Job drawing, mm, ordinate dimensions from the low corner. One solid piece. A direction names the side the tool comes from. Coordinates: 2 decimals unless noted, no trailing zeros. Order: outer loops, then holes, each group sorted by start corner. A loop starts at its lowest first (then second) coordinate and runs counter-clockwise, first axis right, second up. Notation, with made-up numbers: (-27.5, 32.25) - (-2.5, 32.25) arc R36 ccw to (-2.5, 70.25) - close; hole circle Ø7 at (-6, -36). An arc over 180 degrees is marked (long way). Use a Markdown table: item, result. Add a question column.
1) Saw through at A-A on z = 9.5. List the corners of the cut face in (x, y), then the cut area to 3 significant figures.
2) Wall check: L1, parallel to X at y = 0.7, z = 10; L2, parallel to X at y = 0.9, z = 9.5; L3, parallel to Z at x = 32.5, y = 2.25. Give the ranges that are in metal, low to high. Write a range as [from, to].
3) Two-plate mould, pull along Z, no slides. Class the marked faces 1, 2, 3 and 4: +Z half, -Z half, draft (parallel to the pull), parting line (faces both ways), or undercut.
4) Drop flat-ended pins along their axis: P1, Ø1.9, axis at x = 13, z = 24, coming from the +Y side; P2, Ø1, axis at y = 0.5, z = 23.5, coming from the -X side. Give the stop position or say it passes through.
5) Saw through at B-B on x = 13. List the corners of the cut face in (y, z).
6) Saw through at D-D on x = 28. List the corners of the cut face in (y, z).
7) Saw through at C-C on y = 1.9. Count the separate pieces of the cut face and the enclosed holes in it, then the cut area to 3 significant figures.
8) Tool access for the marked faces 5, 6 and 7: list every direction of +Z, -Z, +X, -X, +Y, -Y with a clear straight run to the whole face (end or side of a thin tool).
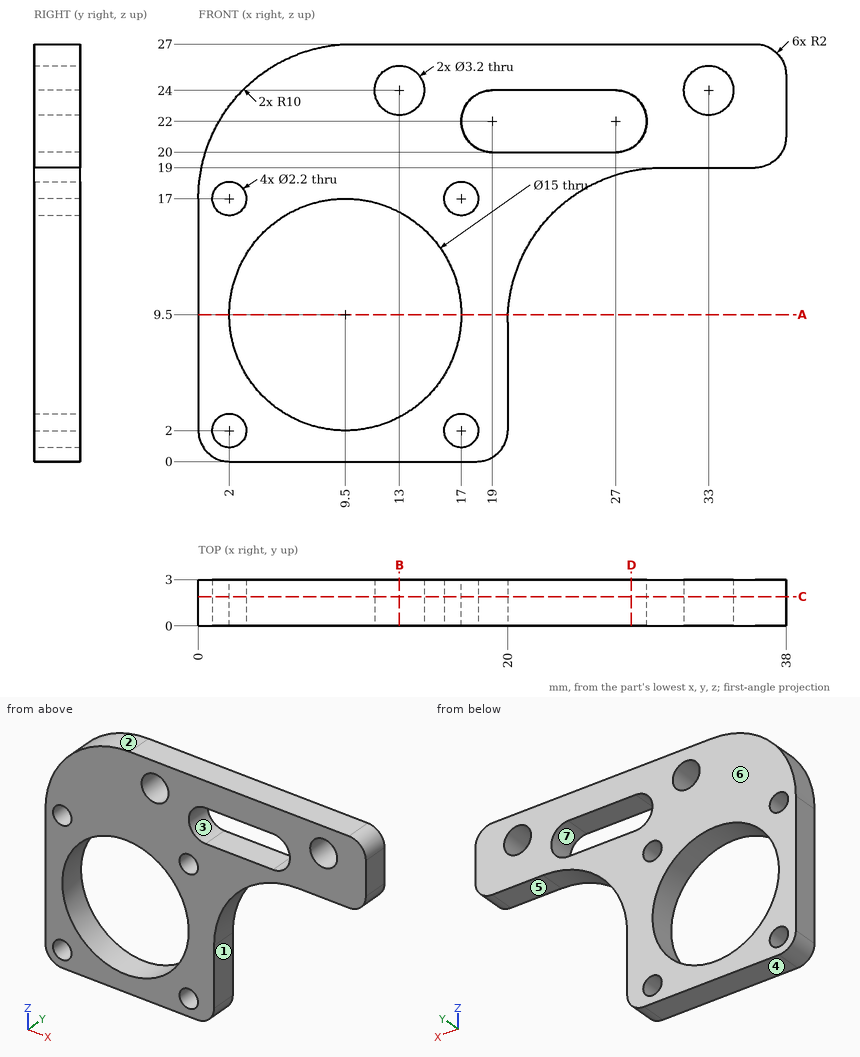
Results are:
| question | item | result |
|---|---|---|
| 1 | outline | (0, 0) - (2, 0) - (2, 3) - (0, 3) - close; (17, 0) - (20.01, 0) - (20.01, 3) - (17, 3) - close |
| 1 | area | 15.0 mm2 |
| 2 | L1 | [0, 2.02], [16.98, 20.05] |
| 2 | L2 | [0, 2], [17, 20.01] |
| 2 | L3 | [19, 22.48], [25.52, 27] |
| 3 | face 1 | draft |
| 3 | face 2 | +Z half |
| 3 | face 3 | undercut |
| 3 | face 4 | -Z half |
| 4 | P1 | through |
| 4 | P2 | x = 2 |
| 5 | outline | (0, 0) - (3, 0) - (3, 2.87) - (0, 2.87) - close; (0, 16.13) - (3, 16.13) - (3, 22.4) - (0, 22.4) - close; (0, 25.6) - (3, 25.6) - (3, 27) - (0, 27) - close |
| 6 | outline | (0, 18.8) - (3, 18.8) - (3, 20.27) - (0, 20.27) - close; (0, 23.73) - (3, 23.73) - (3, 27) - (0, 27) - close |
| 7 | separate pieces | 1 |
| 7 | enclosed holes | 8 |
| 7 | area | 428 mm2 |
| 8 | face 5 | -Z, +X, +Y, -Y |
| 8 | face 6 | +Z, -Z, +X, -X, +Y |
| 8 | face 7 | +Y, -Y |
